Autodesk Inventor part; units mm, degrees
ref_plane "Work Plane1" through (0, 6.5, 0) normal (0, 1, 0) x (1, 0, 0)
ref_plane "YZ Plane" through (0, 0, 0) normal (1, 0, 0) x (0, 1, 0)
ref_plane "XZ Plane" through (0, 0, 0) normal (0, 1, 0) x (-1, 0, 0)
sketch "Sketch1" plane through (0, 0, 0) normal (0, 1, 0) x (-1, 0, 0)
  circle A0 centre (0, 0) radius 7.45
  line L0 (0, 0) -> (-4.32, 12)
  circle A1 centre (-4.32, 12) radius 3.48
  circle A2 centre (-4.32, 12) radius 6.18
  line L1 (-10.5, 28.575) -> (-10.5, -28.575)
  line L2 (7.45, 0) -> (-7.45, 0)
  circle A3 centre (0, 0) radius 10.15
  line L3 (0.5542, 15.7993) -> (8.0054, 6.2399)
  circle A4 centre (-4.32, -12) radius 3.48
  circle A5 centre (-4.32, -12) radius 6.18
  line L4 (0.5542, -15.7993) -> (8.0054, -6.2399)
  point P0 (-10.5, 0)
  point P1 (-10.5, 12)
  point P2 (-10.5, -12)
  dimension "d0" = 14.9
  dimension "d7" = 2.7
  dimension "d1" = 6.96
  dimension "d3" = 10.5
  dimension "d5" = 2.7
  dimension "d6" = 12
extrude "Extrusion1" add sketch "Sketch1" along normal blind 15 contours A0 A2 A3 A5 | A0 L0 A1 A3 A2 | A5 A3 A4 A0 | A0 A2 A3 A1 L0 | A3 A1 A2 | A2 L3 A3 | A5 A3 A2 A0 | A5 A3 A4 | A3 L4 A5 | A5 L1 A2 A3
sketch "Sketch2" plane through (0, 0, 0) normal (0, -1, 0) x (1, 0, 0)
  arc A0 (10.5, 12) -> (-0.5542, 15.7993) centre (4.32, 12) ccw
  line L0 (8.4662, 16.5827) -> (13.8545, 11.7077)
  line L1 (15.5, 8) -> (15.5, 3)
  line L2 (10.5, 12) -> (10.5, -12)
  arc A1 (15.5, 8) -> (13.8545, 11.7077) centre (10.5, 8) ccw
  line L3 (10.5, 0) -> (12.5, 0)
  arc A2 (12.5, 0) -> (15.5, 3) centre (12.5, 3) ccw
  line L4 (10.5, -12) -> (10.5, 12)
  arc A3 (10.5, 12) -> (-0.5542, 15.7993) centre (4.32, 12) ccw
  point P0 (0, 0)
  point P1 (15.5, 0)
  dimension "d10" = 5
  dimension "d11" = 5
  dimension "d12" = 8
  dimension "d13" = 3
  dimension "d14" = 0
extrude "Extrusion2" add sketch "Sketch2" against normal blind 2
ref_plane "Work Plane1" through (0, 6.5, 0) normal (0, 1, 0) x (1, 0, 0)
mirror "Mirror1" about plane through (0, 6.5, 0) normal (0, 1, 0) of "Extrusion2"
fillet "Fillet1" radius 1 6 edges at (6.3287, 15, -17.8444) (-4.2798, 15, -11.0196) (-10.15, 15, 0) (-4.2798, 15, 11.0196) (6.3287, 15, 17.8444) (10.5, 15, 0)
sketch "Sketch3" plane through (0, 15, 0) normal (0, 1, 0) x (1, 0, 0)
  line L0 (-17.025, 1.5) -> (-2.025, 1.5)
  line L1 (-2.025, 1.5) -> (-2.025, -1.5)
  line L2 (-2.025, -1.5) -> (-17.025, -1.5)
  line L3 (-17.025, -1.5) -> (-17.025, 1.5)
  line L4 (-17.025, 1.5) -> (-2.025, -1.5) construction
  line L5 (-2.025, 1.5) -> (-17.025, -1.5) construction
  point P0 (0, 0)
  point P1 (-9.525, 0)
  dimension "d19" = 3
  dimension "d20" = 1.5
  dimension "d21" = 15
extrude "Extrusion3" cut sketch "Sketch3" against normal through all
properties part number "PresaPilotInventorVersion"
Input: part model. Units: mm. Frame: model coordinates. A direction names the side the tool comes from. Round coordinates to 2 decimals unless told otherwise and drop trailing zeros. Loops run counter-clockwise (first coordinate to the right, second up) from the corner with the lowest first, then second, coordinate; pieces in that order, holes last. Notation, with made-up numbers: (81, 76) -> (122, 76) arc R18 ccw to (122, 82) -> close; hole circle Ø10 at (22, 9.5). An arc over 180 degrees is marked (long way). Answer as a JSON object with one key per item and string values. Group by question number.
1) Ray query, L1, parallel to Y at x = 14.25, z = 11; L2, parallel to Z at x = 4.32, y = 8.75; L3, parallel to Z at x = 6.75, y = 4.75. Return the intervals inside material, ascending.
2) Section query A-A on y = 1. Output: boundary loops of the cut face in (x, z).
3) Section query B-B on x = 4.32. Output: boundary loops of the cut face in (y, z), plus the area to 3 significant figures.
4) Pin query (flat end, axial travel): pin 1 (6 mm diameter, centred on y = 4, z = 13.5, fed in from +X); pin 2 (0.6 mm diameter, centred on x = 11.5, y = 12, fed in from -Z); pin 3 (2 mm diameter, centred on x = 11, y = 1, fed in from -Z). Return the tip coordinate at first contact, or that it passes through.
5) Section query C-C on x = 7. State how many separate pieces and enclosed holes the cut face has, plus the area to 3 significant figures.
6) Reachability of faces 1 (the flat face through (11, 1, 0)), 2 (the cylindrical face through (10.199, 14.715, -0.168)), 3 (the flat face through (11.2, 12.01, 14.11)), 4 (the cylindrical face through (6.43, 6.9, 17.81)), 5 (the flat face through (-9, 8, 1.5)) from +Z, -Z, +X, -X, +Y, -Y: full face, straight path, thin tool, end or side. Return the list, or none.
7) Draft query along X for faces 6 (the flat face through (12, 12, 0)), 7 (the cylindrical face through (7.444, 7.395, -0.306)), 8 (the flat face through (15.5, 1, 6)). Return one class per face: +X half, -X half, draft (parallel to the pull), parting line (faces both ways), or undercut.
Reply:
{
 "1": {"L1": "y = 0 to 2, 11 to 13", "L2": "z = -18.18 to -15.48, -8.52 to -6.07, 6.07 to 8.52, 15.48 to 18.18", "L3": "z = -17.68 to -14.49, -9.51 to -3.15, 3.15 to 9.51, 14.49 to 17.68"},
 "2": {"outline": "(-10.04, -1.5) arc R10.15 ccw to (-8.01, -6.24) -> (-0.55, -15.8) arc R6.18 ccw to (10.5, -12) -> (10.5, 0) -> (12.5, 0) arc R3 ccw to (15.5, 3) -> (15.5, 8) arc R5 ccw to (13.85, 11.71) -> (8.47, 16.58) arc R6.18 ccw to (-0.55, 15.8) -> (-8.01, 6.24) arc R10.15 ccw to (-10.04, 1.5) -> (-7.3, 1.5) arc R7.45 cw (long way) to (-7.3, -1.5) -> close; hole circle Ø6.96 at (4.32, -12); hole circle Ø6.96 at (4.32, 12)"},
 "3": {"outline": "(0, -18.18) -> (14, -18.18) arc R1 ccw to (15, -17.18) -> (15, -15.48) -> (0, -15.48) -> close; (0, -8.52) -> (15, -8.52) -> (15, -6.07) -> (0, -6.07) -> close; (0, 6.07) -> (15, 6.07) -> (15, 8.52) -> (0, 8.52) -> close; (0, 15.48) -> (15, 15.48) -> (15, 17.18) arc R1 ccw to (14, 18.18) -> (0, 18.18) -> close", "area": "154 mm2"},
 "4": {"pin 1": "stops at x = 14.29", "pin 2": "stops at z = 0", "pin 3": "stops at z = -14.44"},
 "5": {"separate pieces": "4", "enclosed holes": "0", "area": "317 mm2"},
 "6": {"face 1": "-Z, +X, +Y, -Y", "face 2": "+Z, -Z, +X, +Y", "face 3": "+Z, +X, +Y, -Y", "face 4": "+Z", "face 5": "-X, +Y, -Y"},
 "7": {"face 6": "draft", "face 7": "undercut", "face 8": "+X half"}
}
